Read the model definition and answer for the solid it produces. Units are mm, in the model's axes. A direction names the side the tool comes from. Round coordinates to 2 decimals unless told otherwise and drop trailing zeros. Loops run counter-clockwise (first coordinate to the right, second up) from the corner with the lowest first, then second, coordinate; pieces in that order, holes last. Notation, with made-up numbers: (-37.5, 7.5) - (17.5, 7.5) arc R22 ccw to (17.5, 25.5) - close; hole circle Ø8 at (9, 32). An arc over 180 degrees is marked (long way). Use one line per item in the form item = value. Start each with the question number.
```python
from build123d import *

# Parameters (mm, degrees)
F2_R      = 8.9
F3_DEPTH  = 1.3
F4_R      = 8.9
F5_DEPTH  = 12.8
F7_START  = 5
F7_DEPTH  = 7.05
F9_START  = 5
F8_W      = 5.5
F8_H      = 1.3
F8_H_2    = 3.7
F9_DEPTH  = 3.5
F10_R     = 1.6
F11_DEPTH = 7.05
F12_W     = 3.1
F12_H     = 2.8
F13_DEPTH = 3.5


# Not quite as in the source:
# - a feature of the source that left no trace in its solid (it failed there, or was rolled back) is left out
# - a pattern or mirror of a feature is missing from the dataset's text; its kind, count and spacing are read off the source's solid


with BuildPart() as f1:
    # F0 (on Front) → F1 (revolve)
    with BuildSketch(Plane.XZ):
        Polygon((-12.95, 0), (0, 0), (0, 15), (-12.95, 15), (-12.95, 13.3), (-9.35, 13.3), (-9.35, 6.3), (-12.95, 6.3), (-12.95, 5), (-9.35, 5), (-9.35, 1.3), (-12.95, 1.3), align=None)
    revolve(axis=Axis((0, 0, 7.5), (0, 0, -1)))

    # F2 (on face) → F3 (cut)
    with BuildSketch(Plane(origin=(0, 0, 0), x_dir=(1, 0, 0), z_dir=(0, 0, -1))):
        Circle(F2_R)
    extrude(amount=-F3_DEPTH, mode=Mode.SUBTRACT)

    # F4 (on face) → F5 (cut)
    with BuildSketch(Plane.XY.offset(15)):
        Circle(F4_R)
    extrude(amount=-F5_DEPTH, mode=Mode.SUBTRACT)

    # F6 (on Front) → F7 (join)
    with BuildSketch(Plane.XZ.offset(F7_START)):
        with BuildLine():
            Line((2.75, 6.3), (2.75, 8.15))
            ThreePointArc((2.75, 8.15), (0, 10.9), (-2.75, 8.15))
            Line((-2.75, 8.15), (-2.75, 6.3))
            Line((-2.75, 6.3), (2.75, 6.3))
        make_face()
    f7 = extrude(amount=F7_DEPTH)

    # F7_copies: F7 across plane
    add(f7.mirror(Plane.ZX))

    # F8 (on Front) → F9 (join)
    with BuildSketch(Plane.XZ.offset(F9_START)):
        with BuildLine():
            ThreePointArc((2.75, 8.15), (0, 10.9), (-2.75, 8.15))
            Line((-2.75, 8.15), (-2.75, 6.3))
            Line((-2.75, 6.3), (2.75, 6.3))
            Line((2.75, 6.3), (2.75, 8.15))
        make_face()
        with Locations((0, 5.65)):
            Rectangle(F8_W, F8_H)
        with Locations((0, 3.15)):
            Rectangle(F8_W, F8_H_2)
    f9 = extrude(amount=F9_DEPTH)

    # F9_copies: F9 across plane
    add(f9.mirror(Plane.ZX))

    # F10 (on face) → F11 (cut, through all)
    with BuildSketch(Plane.XZ.offset(12.05)):
        with Locations((0, 8.15)):
            Circle(F10_R)
    f11 = extrude(amount=-F11_DEPTH, mode=Mode.SUBTRACT)

    # F11_copies: F11 across plane
    add(f11.mirror(Plane.ZX), mode=Mode.SUBTRACT)

    # F12 (on face) → F13 (cut)
    with BuildSketch(Plane(origin=(0, 0, 1.3), x_dir=(1, 0, 0), z_dir=(0, 0, -1))):
        with Locations((0, 7.3639888179)):
            Rectangle(F12_W, F12_H)
    f13 = extrude(amount=-F13_DEPTH, mode=Mode.SUBTRACT)

    # F13_copies: F13 across plane
    add(f13.mirror(Plane.ZX), mode=Mode.SUBTRACT)


solid = f1.part
```
1) Straight lines are drawn through the part: line 1 (Z direction, x = -11.5, y = 3); line 2 (Z direction, x = 0, y = -10.5); line 3 (Y direction, x = 0, z = 0.95). For each, find the intervals that lie inside material, in ascending order. Write a range as from..to.
2) Flat-ended cylindrical pins translate along their axes: pin 1 (4 mm diameter, centred on x = 5, z = 4.5, fed in from +Y); pin 2 (2 mm diameter, centred on x = 0, y = -7, fed in from +Z); pin 3 (1.4 mm diameter, centred on x = 0, z = 9.5, fed in from -Y). Find the tip coordinate at first contact, or state that the pin passes through.
3) A cutting plane is placed at B-B on y = 0. Write down the section's boundary in (x, z), plus the area to 3 significant figures.
4) A cutting plane is placed at D-D on x = -4. Write down the section's boundary in (y, z), plus the area to 3 significant figures.
5) A cutting plane is placed at A-A on z = 3.25. Write down the section's boundary in (x, y).
6) For faces 4 (the cylindrical face through (0.1, -10.5, 10.9)), 5 (the flat face through (0, 5.964, 3)), 6 (the flat face through (2.75, -7, 5)), 7 (the cylindrical face through (2.027, -9.128, 3.124)), determine the directions among +Z, -Z, +X, -X, +Y, -Y from which every point of the face is accessible in a straight line to the end or side of a thin tool.
7) Determine the mould class of faces 1 (the flat face through (-2.75, 10, 7)), 2 (the cylindrical face through (2.81, -12.64, 0.64)), 3 (the flat face through (1.55, -7, 3)) for opening direction Y: +Y half, -Y half, draft (parallel to the pull), parting line (faces both ways), or undercut.
8) A cutting plane is placed at C-C on z = 5.5. Write down the section's boundary in (x, y).
Checks:
q1.line_1 = 0..1.3, 5..6.3, 13.3..15
q1.line_2 = 0..1.3, 5..6.55, 9.75..10.9, 13.3..15
q1.line_3 = -12.95..-8.9, 8.9..12.95
q2.pin_1 = 12.58
q2.pin_2 = 10.9
q2.pin_3 = -12.05
q3.outline = (-12.95, 0) - (-8.9, 0) - (-8.9, 1.3) - (8.9, 1.3) - (8.9, 0) - (12.95, 0) - (12.95, 1.3) - (9.35, 1.3) - (9.35, 5) - (12.95, 5) - (12.95, 6.3) - (9.35, 6.3) - (9.35, 13.3) - (12.95, 13.3) - (12.95, 15) - (8.9, 15) - (8.9, 2.2) - (-8.9, 2.2) - (-8.9, 15) - (-12.95, 15) - (-12.95, 13.3) - (-9.35, 13.3) - (-9.35, 6.3) - (-12.95, 6.3) - (-12.95, 5) - (-9.35, 5) - (-9.35, 1.3) - (-12.95, 1.3) - close
q3.area = 60.5 mm²
q4.outline = (-12.32, 0) - (-7.95, 0) - (-7.95, 1.3) - (7.95, 1.3) - (7.95, 0) - (12.32, 0) - (12.32, 1.3) - (8.45, 1.3) - (8.45, 5) - (12.32, 5) - (12.32, 6.3) - (8.45, 6.3) - (8.45, 13.3) - (12.32, 13.3) - (12.32, 15) - (7.95, 15) - (7.95, 2.2) - (-7.95, 2.2) - (-7.95, 15) - (-12.32, 15) - (-12.32, 13.3) - (-8.45, 13.3) - (-8.45, 6.3) - (-12.32, 6.3) - (-12.32, 5) - (-8.45, 5) - (-8.45, 1.3) - (-12.32, 1.3) - close
q4.area = 62.6 mm²
q5.outline = circle Ø18.7 at (0, 0); hole (-2.75, -8.46) - (-2.75, -5) - (2.75, -5) - (2.75, -8.46) arc R8.9 ccw to (2.75, 8.46) - (2.75, 5) - (-2.75, 5) - (-2.75, 8.46) arc R8.9 ccw to start; hole (-2.64, -8.5) arc R8.9 ccw to (2.64, -8.5) - (1.55, -8.5) - (1.55, -5.96) - (-1.55, -5.96) - (-1.55, -8.5) - close; hole (-2.64, 8.5) - (-1.55, 8.5) - (-1.55, 5.96) - (1.55, 5.96) - (1.55, 8.5) - (2.64, 8.5) arc R8.9 ccw to start
q6.face_4 = -Y
q6.face_5 = -Z
q6.face_6 = +Z
q6.face_7 = none
q7.face_1 = draft
q7.face_2 = parting line
q7.face_3 = undercut
q8.outline = circle Ø25.9 at (0, 0); hole (-2.75, -8.46) - (-2.75, -5) - (2.75, -5) - (2.75, -8.46) arc R8.9 ccw to (2.75, 8.46) - (2.75, 5) - (-2.75, 5) - (-2.75, 8.46) arc R8.9 ccw to start; hole (-2.64, -8.5) arc R8.9 ccw to (2.64, -8.5) - close; hole (-2.64, 8.5) - (2.64, 8.5) arc R8.9 ccw to start
